Drawing for the job (mm, zero at the part's lowest x, y, z). A direction names the side the tool comes from. Coordinates: 2 decimals unless noted, no trailing zeros. Loops run counter-clockwise (first coordinate to the right, second up) from the corner with the lowest first, then second, coordinate; pieces in that order, holes last. Notation, with made-up numbers: (-4.5, 38) -> (51.5, 38) arc R21 ccw to (51.5, 73) -> close; hole circle Ø2 at (42, 58.5). An arc over 180 degrees is marked (long way). Write item = value, one per line. Start each with the question number.
(1) Band-saw the part on A-A (z = 39.5). Write the cut outline in (x, y).
(2) Band-saw the part on D-D (z = 70). Write the cut outline in (x, y), and give its area (3 significant figures).
(3) Pull direction Y, two halves, no side cores. Call the marked faces 1, 2 and 3: +Y half, -Y half, draft (parallel to the pull), parting line (faces both ways), or undercut.
(4) Tool access for the marked faces 4, 5 and 6: list every direction of +Z, -Z, +X, -X, +Y, -Y with a clear straight run to the whole face (end or side of a thin tool).
(5) Drill centre lines: line 1 (Y direction, x = 79, z = 38); line 2 (X direction, y = 116, z = 75); line 3 (Z direction, x = 50, y = 87.5). Where is each one in solid material? Low to high. Write a range as from..to.
(6) Flat gauge pins, fed straight in: P1, Ø4, axis at y = 120, z = 40.5, coming from the -X side; P2, Ø5, axis at x = 26.5, z = 50.5, coming from the -Y side; P3, Ø6.5, axis at y = 226.5, z = 58.5, coming from the +X side. Where does each tip first touch, or does it go through?
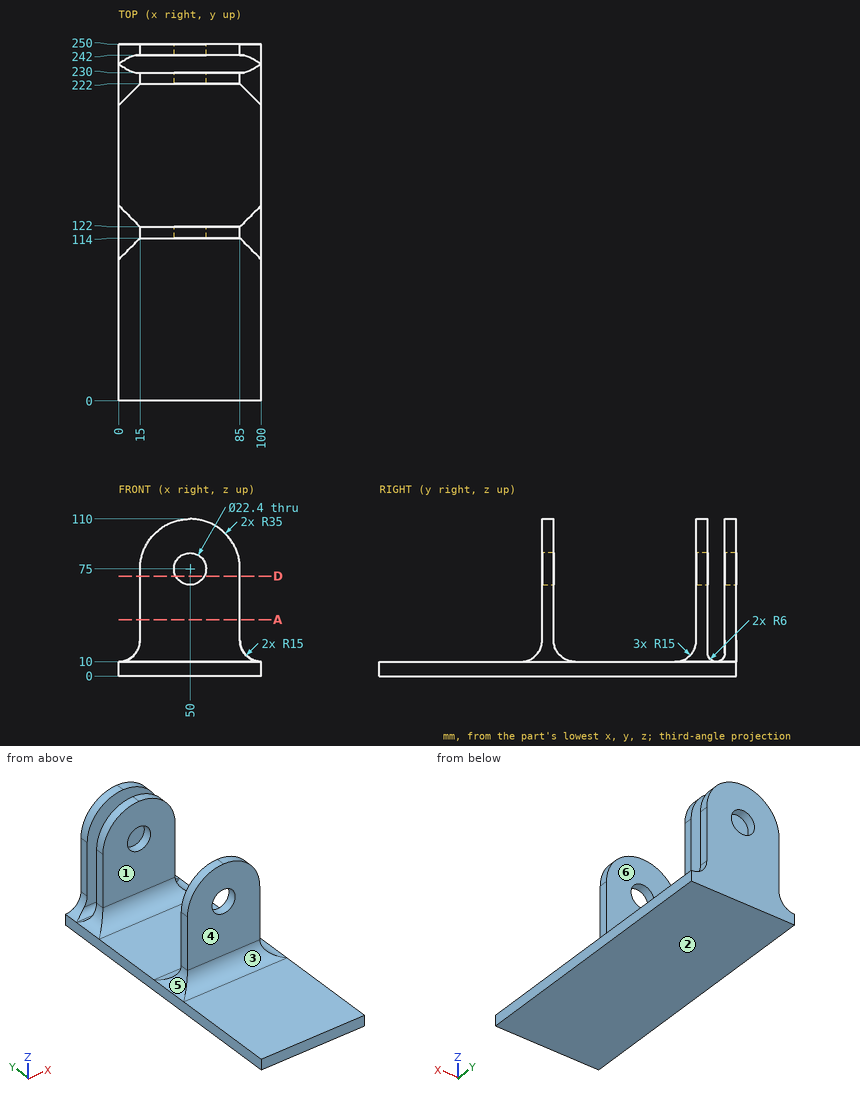
Findings below:
q1.outline = (15, 114) -> (85, 114) -> (85, 122) -> (15, 122) -> close; (15, 222) -> (85, 222) -> (85, 230) -> (15, 230) -> close; (15, 242) -> (85, 242) -> (85, 250) -> (15, 250) -> close
q2.outline = (15, 114) -> (39.98, 114) -> (39.98, 122) -> (15, 122) -> close; (15, 222) -> (39.98, 222) -> (39.98, 230) -> (15, 230) -> close; (15, 242) -> (39.98, 242) -> (39.98, 250) -> (15, 250) -> close; (60.02, 114) -> (85, 114) -> (85, 122) -> (60.02, 122) -> close; (60.02, 222) -> (85, 222) -> (85, 230) -> (60.02, 230) -> close; (60.02, 242) -> (85, 242) -> (85, 250) -> (60.02, 250) -> close
q2.area = 1,200 mm²
q3.face_1 = undercut
q3.face_2 = draft
q3.face_3 = -Y half
q4.face_4 = +Z, +X, -X, -Y
q4.face_5 = +Z, -X, +Y, -Y
q4.face_6 = +Z, +X, -X
q5.line_1 = 114..122, 222..230, 242..250
q5.line_2 = 15..38.8, 61.2..85
q5.line_3 = 0..10
q6.P1 = 15
q6.P2 = 114
q6.P3 = 85
